from build123d import *

# Parameters (mm, degrees)
ESTRUSIONE_ESTRUSIONE1_DEPTH = 2
SCHIZZO2_R                   = 1.65
TAGLIO_ESTRUSIONE1_DEPTH     = 2
SCHIZZO3_R                   = 12.5
TAGLIO_ESTRUSIONE2_DEPTH     = 2
SCHIZZO4_R                   = 2
TAGLIO_ESTRUSIONE3_DEPTH     = 2


with BuildPart() as part:
    # Schizzo1 → Estrusione-Estrusione1 (new body)
    with BuildSketch(Plane.XY):
        with BuildLine():
            Line((21, 0), (21, -60))
            Line((21, -60), (-21, -60))
            Line((-21, -60), (-21, 0))
            ThreePointArc((-21, 0), (0, 21), (21, 0))
        make_face()
    extrude(amount=ESTRUSIONE_ESTRUSIONE1_DEPTH)

    # Schizzo2 → Taglio-Estrusione1 (cut)
    with BuildSketch(Plane.XY.offset(2)):
        with Locations((-18, 0)):
            Circle(SCHIZZO2_R)
        with Locations((18, 0)):
            Circle(SCHIZZO2_R)
        with Locations((0, 18)):
            Circle(SCHIZZO2_R)
        with Locations((0, -18)):
            Circle(SCHIZZO2_R)
    extrude(amount=-TAGLIO_ESTRUSIONE1_DEPTH, mode=Mode.SUBTRACT)

    # Schizzo3 → Taglio-Estrusione2 (cut)
    with BuildSketch(Plane.XY.offset(2)):
        Circle(SCHIZZO3_R)
    extrude(amount=-TAGLIO_ESTRUSIONE2_DEPTH, mode=Mode.SUBTRACT)

    # Schizzo4 → Taglio-Estrusione3 (cut)
    with BuildSketch(Plane.XY.offset(2)):
        with Locations((-10, -29)):
            Circle(SCHIZZO4_R)
        with Locations((10, -29)):
            Circle(SCHIZZO4_R)
        with Locations((10, -49)):
            Circle(SCHIZZO4_R)
        with Locations((-10, -49)):
            Circle(SCHIZZO4_R)
    extrude(amount=-TAGLIO_ESTRUSIONE3_DEPTH, mode=Mode.SUBTRACT)


solid = part.part
Input: part model. Units: mm. Frame: model coordinates. Coordinates: 2 decimals unless noted, no trailing zeros. Order: outer loops, then holes, each group sorted by start corner. A loop starts at its lowest first (then second) coordinate and runs counter-clockwise, first axis right, second up. Notation, with made-up numbers: M 21.25,11 L 47.25,11 A25 cw 47.25,25 Z; hole C 69.25,13.5 d9. An arc over 180 degrees is marked long. Write item = value, one per line. Start each with the question number.
(1) First-contact query: P1, Ø4, axis at x = -18, y = 0, coming from the -Z side; P2, Ø2.5, axis at x = 0, y = 18, coming from the +Z side. Flat tips, straight axial feed; report the tip coordinate or a pass-through.
(2) Line query: line 1 along Y through (x, z) = (0, 1.5); line 2 along Y through (x, z) = (9, 1.2); line 3 along X through (y, z) = (1.5, 0.5). Output: solid intervals per line, ascending. Write a range as [from, to].
(3) Pull-direction query (X, two-part tool) for faces 1 (the flat face through (0, -60, 1)), 2 (the cylindrical face through (-10, -31, 1)), 3 (the cylindrical face through (0, 21, 1)); classes: released by +X, released by -X, zero draft, split by the parting line, or undercut.
(4) Section C-C on x = 0. Output: boundary loops of the cut face in (y, z), and give its area (3 significant figures).
(5) Section D-D on z = 1.05. Give the number of separate pieces and of enclosed holes in the cut face, and give its area (3 significant figures).
(6) Section B-B on y = -29. Output: boundary loops of the cut face in (x, z), and give its area (3 significant figures).
(7) Section A-A on y = -18. Output: boundary loops of the cut face in (x, z), and give its area (3 significant figures).
Result set:
q1.P1 = 0
q1.P2 = through
q2.line_1 = [-60, -19.65], [-16.35, -12.5], [12.5, 16.35], [19.65, 21]
q2.line_2 = [-60, -50.73], [-47.27, -30.73], [-27.27, -8.67], [8.67, 18.97]
q2.line_3 = [-20.95, -18.69], [-17.31, -12.41], [12.41, 17.31], [18.69, 20.95]
q3.face_1 = zero draft
q3.face_2 = undercut
q3.face_3 = split by the parting line
q4.outline = M -60,0 L -19.65,0 L -19.65,2 L -60,2 Z; M -16.35,0 L -12.5,0 L -12.5,2 L -16.35,2 Z; M 12.5,0 L 16.35,0 L 16.35,2 L 12.5,2 Z; M 19.65,0 L 21,0 L 21,2 L 19.65,2 Z
q4.area = 98.8 mm²
q5.separate_pieces = 1
q5.enclosed_holes = 9
q5.area = 2,640 mm²
q6.outline = M -21,0 L -12,0 L -12,2 L -21,2 Z; M -8,0 L 8,0 L 8,2 L -8,2 Z; M 12,0 L 21,0 L 21,2 L 12,2 Z
q6.area = 68.0 mm²
q7.outline = M -21,0 L -1.65,0 L -1.65,2 L -21,2 Z; M 1.65,0 L 21,0 L 21,2 L 1.65,2 Z
q7.area = 77.4 mm²
